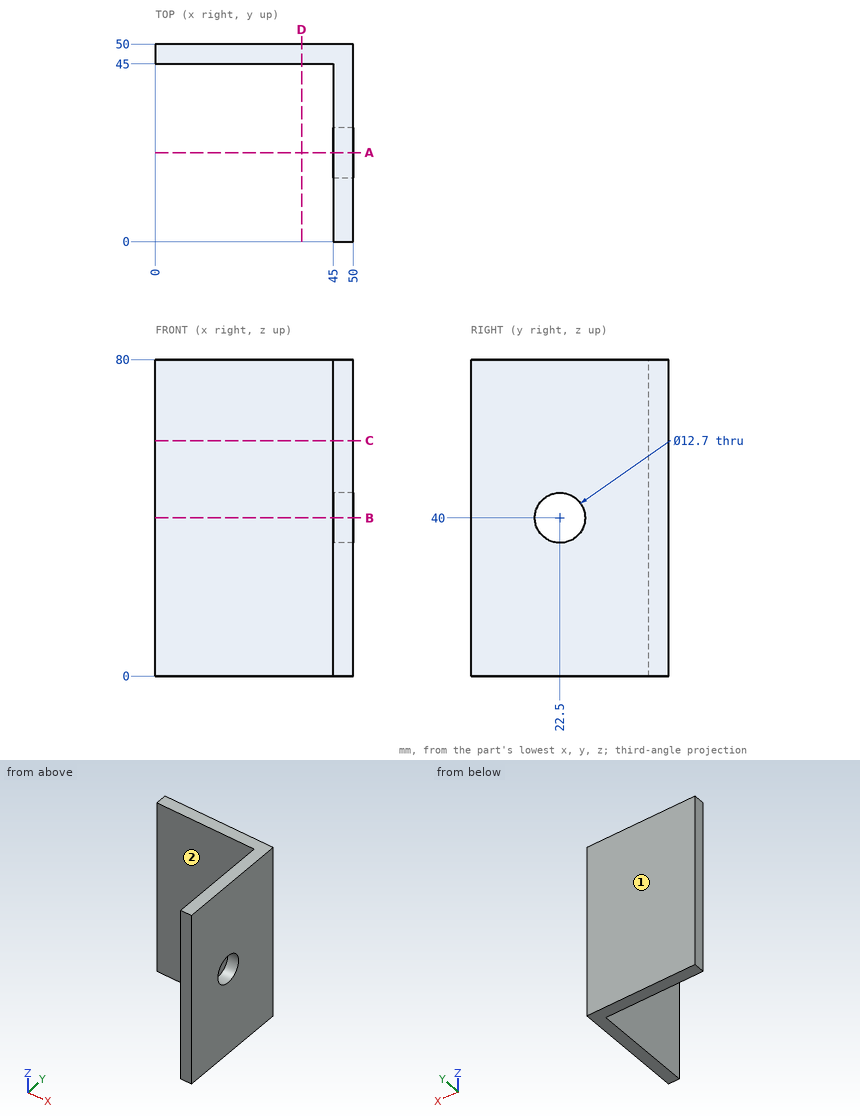
Geometry check sheet. Reference: drawing and pictorial views, mm from the part's lowest x, y, z. A direction names the side the tool comes from. Round coordinates to 2 decimals unless told otherwise and drop trailing zeros. Loops run counter-clockwise (first coordinate to the right, second up) from the corner with the lowest first, then second, coordinate; pieces in that order, holes last. Notation, with made-up numbers: (25, -1) -> (73, -1) arc R28 ccw to (73, 17) -> close; hole circle Ø3 at (-1.5, 47). An arc over 180 degrees is marked (long way). Answer as a JSON object with one key per item and string values.
Q1. Go/stop test with flat-tipped pins: P1, Ø22.5, axis at y = 23.5, z = 26, coming from the -X side; P2, Ø13.5, axis at x = 20, z = 55.5, coming from the -Y side. Record where each tip stops, or that it passes through.
Data:
{"P1": "stops at x = 45", "P2": "stops at y = 45"}
Q2. Section check C-C (z = 59.5). Record the boundary of the cut face in (x, y).
Data:
{"outline": "(0, 45) -> (45, 45) -> (45, 0) -> (50, 0) -> (50, 50) -> (0, 50) -> close"}
Q3. Section check A-A (y = 22.5). Record the boundary of the cut face in (x, z).
Data:
{"outline": "(45, 0) -> (50, 0) -> (50, 33.65) -> (45, 33.65) -> close; (45, 46.35) -> (50, 46.35) -> (50, 80) -> (45, 80) -> close"}
Q4. Section check B-B (z = 40). Record the boundary of the cut face in (x, y).
Data:
{"outline": "(0, 45) -> (45, 45) -> (45, 28.85) -> (50, 28.85) -> (50, 50) -> (0, 50) -> close; (45, 0) -> (50, 0) -> (50, 16.15) -> (45, 16.15) -> close"}
Q5. Section check D-D (x = 37). Record the boundary of the cut face in (y, z).
Data:
{"outline": "(45, 0) -> (50, 0) -> (50, 80) -> (45, 80) -> close"}
Q6. Scan lines: line 1 (Z direction, x = 48.9, y = 22.5); line 2 (Y direction, x = 21, z = 66.5). Record each from-to range of solid material in increasing order. Write a range as from..to.
Data:
{"line 1": "z = 0..33.65, 46.35..80", "line 2": "y = 45..50"}
Q7. Access from +Z, -Z, +X, -X, +Y, -Y to the whole of each face (thin tool, end or side, straight path). Record for the marked faces 1 and 2.
Data:
{"face 1": "+Z, -Z, +X, -X, +Y", "face 2": "+Z, -Z, -X, -Y"}
